Work out the finished part from the listing and answer in its coordinate system (mm). Face numbers are marked on the shaded views. A direction names the side the tool comes from. Round coordinates to 2 decimals unless told otherwise and drop trailing zeros. Loops run counter-clockwise (first coordinate to the right, second up) from the corner with the lowest first, then second, coordinate; pieces in that order, holes last. Notation, with made-up numbers: (-3, 38.25) - (32, 38.25) arc R19 ccw to (32, 45.25) - close; hole circle Ø10 at (87, 38). An arc over 180 degrees is marked (long way). Return JSON: item names as keys, results as strings.
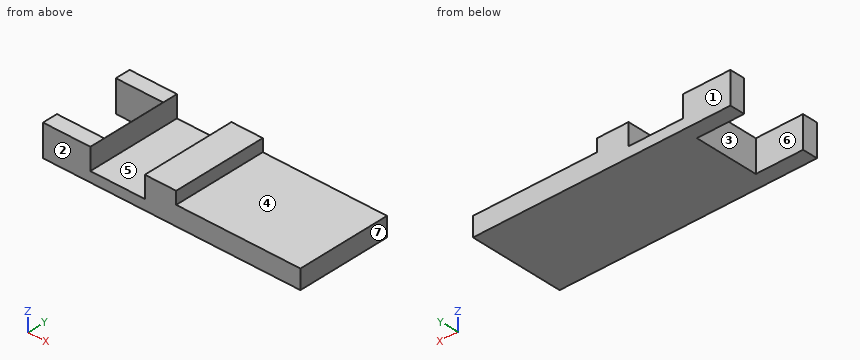
from build123d import *

# Parameters (mm, degrees)
F1_DEPTH = 25.4
F2_W     = 16.138606
F2_H     = 17.284541
F3_DEPTH = 8.543421


with BuildPart() as f1:
    # F0 (on Front) → F1 (new body)
    with BuildSketch(Plane.XZ):
        Polygon((-36.821757, 8.542421), (-49.570106, 8.542421), (-49.570106, 0), (19.731788, 0), (19.731788, 5.173579), (-13.715999, 5.173579), (-13.715999, 8.542421), (-22.151655, 8.542421), (-22.151655, 2.737268), (-36.821757, 2.737268), align=None)
    extrude(amount=F1_DEPTH)

    # F2 (on Top) → F3 (cut, through all)
    with BuildSketch(Plane.XY):
        with Locations((-44.908296, -12.673702)):
            Rectangle(F2_W, F2_H)
    extrude(amount=F3_DEPTH, mode=Mode.SUBTRACT)


solid = f1.part
1) Section A-A (z = 4.25) is taken. Give the vertices of the cut face in (x, y).
Verdict:
{"outline": "(-49.57, -25.4) - (-36.82, -25.4) - (-36.82, 0) - (-49.57, 0) - (-49.57, -4.03) - (-36.84, -4.03) - (-36.84, -21.32) - (-49.57, -21.32) - close; (-22.15, -25.4) - (19.73, -25.4) - (19.73, 0) - (-22.15, 0) - close"}
2) Section C-C (z = 0.75) is taken. Give the vertices of the cut face in (x, y), and give its area (3 significant figures).
Verdict:
{"outline": "(-49.57, -25.4) - (19.73, -25.4) - (19.73, 0) - (-49.57, 0) - (-49.57, -4.03) - (-36.84, -4.03) - (-36.84, -21.32) - (-49.57, -21.32) - close", "area": "1,540 mm2"}
3) Section D-D (x = -12) is taken. Give the vertices of the cut face in (y, z).
Verdict:
{"outline": "(-25.4, 0) - (0, 0) - (0, 5.17) - (-25.4, 5.17) - close"}
4) Flat-ended cylindrical pins translate along their axes: pin 1 (1.5 mm diameter, centred on y = -3.5, z = 6, fed in from +X); pin 2 (7.5 mm diameter, centred on x = -3.5, y = -9.5, fed in from +Z); pin 3 (3 mm diameter, centred on y = -7.5, z = 1, fed in from -X). Find the tip coordinate at first contact, or state that the pin passes through.
Verdict:
{"pin 1": "stops at x = -13.72", "pin 2": "stops at z = 5.17", "pin 3": "stops at x = -36.84"}
5) Find the intervals of material crossed by L1, parallel to X at y = -23.75, z = 7.75; L2, parallel to Y at x = -42, z = 4; L3, parallel to Z at x = -11.5, y = -13.5, in increasing order.
Verdict:
{"L1": "x = -49.57 to -36.82, -22.15 to -13.72", "L2": "y = -25.4 to -21.32, -4.03 to 0", "L3": "z = 0 to 5.17"}
6) A tool of negligible diameter and unlimited length cuts with its end or side. For the marked faces 5, 6 and 7, from which of +Z, -Z, +X, -X, +Y, -Y can it reach the whole face along a straight path? Write none if from no direction.
Verdict:
{"face 5": "+Z, +Y, -Y", "face 6": "+Z, -Z, -X", "face 7": "+Z, -Z, +X, +Y, -Y"}
7) Determine the mould class of the marked faces 1, 2, 3 and 4 for opening direction Y: pulls with the +Y half, pulls with the -Y half, needs draft (parallel to the pull), parting line crosses it, or undercut.
Verdict:
{"face 1": "pulls with the +Y half", "face 2": "pulls with the -Y half", "face 3": "undercut", "face 4": "needs draft"}
